Read the model definition and answer for the solid it produces. Units are mm, in the model's axes. A direction names the side the tool comes from. Coordinates: 2 decimals unless noted, no trailing zeros. Loops run counter-clockwise (first coordinate to the right, second up) from the corner with the lowest first, then second, coordinate; pieces in that order, holes last. Notation, with made-up numbers: (74, 76.25) - (115, 76.25) arc R30 ccw to (115, 112.25) - close; hole circle Ø10 at (-11.5, 47.5). An arc over 180 degrees is marked (long way). Use one line per item in the form item = value.
Autodesk Inventor part; units mm, degrees
ref_plane "YZ Plane" through (0, 0, 0) normal (1, 0, 0) x (0, 1, 0)
ref_plane "XZ Plane" through (0, 0, 0) normal (0, 1, 0) x (-1, 0, 0)
ref_plane "XY Plane" through (0, 0, 0) normal (0, 0, 1) x (1, 0, 0)
sketch "Sketch1" plane through (0, 0, 0) normal (0, 0, 1) x (1, 0, 0)
  line L0 (-11, 11) -> (11, 11)
  line L1 (11, 11) -> (11, -11)
  line L2 (11, -11) -> (-11, -11)
  line L3 (-11, -11) -> (-11, 11)
  point P0 (0, 0)
  point P1 (-11, 0)
  point P2 (0, 11)
  dimension "d0" = 22
extrude "Extrusion1" add sketch "Sketch1" along normal blind 3.4
sketch "Sketch2" plane through (0, 0, 3.4) normal (0, 0, 1) x (1, 0, 0)
  circle A0 centre (0, 0) radius 8.98 construction
  line L0 (-6.3498, 6.3498) -> (6.3498, 6.3498) construction
  line L1 (6.3498, 6.3498) -> (6.3498, -6.3498) construction
  line L2 (6.3498, -6.3498) -> (-6.3498, -6.3498) construction
  line L3 (-6.3498, -6.3498) -> (-6.3498, 6.3498) construction
  line L4 (-3.4498, 8.0241) -> (-3.4498, 4.6755)
  line L5 (-3.4498, 4.6755) -> (-6.3498, 3.0012)
  line L6 (-6.3498, 3.0012) -> (-9.2498, 4.6755)
  line L7 (-9.2498, 4.6755) -> (-9.2498, 8.0241)
  line L8 (-9.2498, 8.0241) -> (-6.3498, 9.6985)
  line L9 (-6.3498, 9.6985) -> (-3.4498, 8.0241)
  line L10 (9.2498, 8.0241) -> (9.2498, 4.6755)
  line L11 (9.2498, 4.6755) -> (6.3498, 3.0012)
  line L12 (6.3498, 3.0012) -> (3.4498, 4.6755)
  line L13 (3.4498, 4.6755) -> (3.4498, 8.0241)
  line L14 (3.4498, 8.0241) -> (6.3498, 9.6985)
  line L15 (6.3498, 9.6985) -> (9.2498, 8.0241)
  line L16 (9.2498, -4.6755) -> (9.2498, -8.0241)
  line L17 (9.2498, -8.0241) -> (6.3498, -9.6985)
  line L18 (6.3498, -9.6985) -> (3.4498, -8.0241)
  line L19 (3.4498, -8.0241) -> (3.4498, -4.6755)
  line L20 (3.4498, -4.6755) -> (6.3498, -3.0012)
  line L21 (6.3498, -3.0012) -> (9.2498, -4.6755)
  line L22 (-6.3498, -3.0012) -> (-3.4498, -4.6755)
  line L23 (-3.4498, -4.6755) -> (-3.4498, -8.0241)
  line L24 (-3.4498, -8.0241) -> (-6.3498, -9.6985)
  line L25 (-6.3498, -9.6985) -> (-9.2498, -8.0241)
  line L26 (-9.2498, -8.0241) -> (-9.2498, -4.6755)
  line L27 (-9.2498, -4.6755) -> (-6.3498, -3.0012)
  point P0 (6.3498, -6.3498)
  dimension "d3" = 17.96
  dimension "d4" = 5.8
extrude "Extrusion2" cut sketch "Sketch2" against normal blind 4
sketch "Sketch3" plane through (0, 0, 0) normal (0, 0, -1) x (-1, 0, 0)
  line L0 (-3.4498, -4.6755) -> (-3.4498, -8.0241)
  line L1 (-3.4498, -8.0241) -> (-6.3498, -9.6985)
  line L2 (-6.3498, -9.6985) -> (-9.2498, -8.0241)
  line L3 (-9.2498, -8.0241) -> (-9.2498, -4.6755)
  line L4 (-9.2498, -4.6755) -> (-6.3498, -3.0012)
  line L5 (-6.3498, -3.0012) -> (-3.4498, -4.6755)
  line L6 (-3.4498, 8.0241) -> (-3.4498, 4.6755)
  line L7 (-3.4498, 4.6755) -> (-6.3498, 3.0012)
  line L8 (-6.3498, 3.0012) -> (-9.2498, 4.6755)
  line L9 (-9.2498, 4.6755) -> (-9.2498, 8.0241)
  line L10 (-9.2498, 8.0241) -> (-6.3498, 9.6985)
  line L11 (-6.3498, 9.6985) -> (-3.4498, 8.0241)
  line L12 (9.2498, -8.0241) -> (6.3498, -9.6985)
  line L13 (6.3498, -9.6985) -> (3.4498, -8.0241)
  line L14 (3.4498, -8.0241) -> (3.4498, -4.6755)
  line L15 (3.4498, -4.6755) -> (6.3498, -3.0012)
  line L16 (6.3498, -3.0012) -> (9.2498, -4.6755)
  line L17 (9.2498, -4.6755) -> (9.2498, -8.0241)
  line L18 (9.2498, 8.0241) -> (9.2498, 4.6755)
  line L19 (9.2498, 4.6755) -> (6.3498, 3.0012)
  line L20 (6.3498, 3.0012) -> (3.4498, 4.6755)
  line L21 (3.4498, 4.6755) -> (3.4498, 8.0241)
  line L22 (3.4498, 8.0241) -> (6.3498, 9.6985)
  line L23 (6.3498, 9.6985) -> (9.2498, 8.0241)
  line L24 (11, -11) -> (-11, -11)
  line L25 (11, 11) -> (11, -11)
  line L26 (-11, 11) -> (11, 11)
  line L27 (-11, -11) -> (-11, 11)
  circle A0 centre (6.3498, 6.3498) radius 1.75
  circle A1 centre (6.3498, -6.3498) radius 1.75
  circle A2 centre (-6.3498, -6.3498) radius 1.75
  circle A3 centre (-6.3498, 6.3498) radius 1.75
  point P0 (0, 0)
  point P1 (9.2498, -6.3498)
  point P2 (-3.4498, -6.3498)
  point P3 (-3.4498, 6.3498)
  point P4 (9.2498, 6.3498)
  dimension "d7" = 3.5
extrude "Extrusion3" add sketch "Sketch3" against normal blind 1 contours L0 L1 L2 L3 L4 L5 | L6 L7 L8 L9 L10 L11 | L12 L13 L14 L15 L16 L17 | L18 L19 L20 L21 L22 L23
fillet "Fillet1" radius 2 4 edges at (11, 11, 1.7) (-11, 11, 1.7) (11, -11, 1.7) (-11, -11, 1.7)
sketch "Sketch4" plane through (0, 0, 3.4) normal (0, 0, 1) x (1, 0, 0)
  circle A0 centre (0, 0) radius 4.1
  dimension "d11" = 8.2
extrude "Extrusion4" cut sketch "Sketch4" against normal through all
chamfer "Chamfer1" distance 0.4 angle 45 16 edges at (0, 11, 0) (-10.4142, 10.4142, 0) (-11, 0, 0) (-10.4142, -10.4142, 0) (0, -11, 0) (10.4142, -10.4142, 0) (11, 0, 0) (10.4142, 10.4142, 0) (0, 11, 3.4) (-10.4142, 10.4142, 3.4) (-11, 0, 3.4) (-10.4142, -10.4142, 3.4) (0, -11, 3.4) (10.4142, -10.4142, 3.4) (11, 0, 3.4) (10.4142, 10.4142, 3.4)
chamfer "Chamfer2" distance 0.4 angle 45 2 edges at (-4.1, 0, 0) (-4.1, 0, 3.4)
properties part number "bnc-nut-support" material "ABS Plastic"
Item 1: The part is cut by section A-A on y = 0. Give the vertices of the cut face in (x, z).
Results below:
outline = (-11, 0.4) - (-10.6, 0) - (-4.5, 0) - (-4.1, 0.4) - (-4.1, 3) - (-4.5, 3.4) - (-10.6, 3.4) - (-11, 3) - close; (4.1, 0.4) - (4.5, 0) - (10.6, 0) - (11, 0.4) - (11, 3) - (10.6, 3.4) - (4.5, 3.4) - (4.1, 3) - close
Item 2: Find the intervals of material crossed by L1, parallel to X at y = 7, z = 2.8; L2, parallel to X at y = -6.5, z = 0.85; L3, parallel to Y at x = -6, z = 2.45, in increasing order.
Results below:
L1 = -11 to -9.25, -3.45 to 3.45, 9.25 to 11
L2 = -11 to -8.09, -4.61 to 4.61, 8.09 to 11
L3 = -11 to -9.5, -3.2 to 3.2, 9.5 to 11
Item 3: The part is cut by section D-D on y = 7. Give the vertices of the cut face in (x, z).
Results below:
outline = (-11, 0.4) - (-10.6, 0) - (-7.97, 0) - (-7.97, 1) - (-9.25, 1) - (-9.25, 3.4) - (-10.6, 3.4) - (-11, 3) - close; (-4.73, 0) - (4.73, 0) - (4.73, 1) - (3.45, 1) - (3.45, 3.4) - (-3.45, 3.4) - (-3.45, 1) - (-4.73, 1) - close; (7.97, 0) - (10.6, 0) - (11, 0.4) - (11, 3) - (10.6, 3.4) - (9.25, 3.4) - (9.25, 1) - (7.97, 1) - close
Item 4: The part is cut by section C-C on z = 2.5. Count the separate pieces of the cut face and the enclosed holes in it, plus the area to 3 significant figures.
Results below:
separate_pieces = 1
enclosed_holes = 5
area = 311 mm²
Item 5: For a pull along Y with two mould halves and no side action, classify faces 3 (the flat face through (-4.88, -8.85, 2.22)), 4 (the flat face through (-7.779, 3.827, 2.217)), 5 (the flat face through (11, 0, 2)), 6 (the conical face through (10.225, -10.199, 3.286)) as +Y half, -Y half, draft (parallel to the pull), parting line (faces both ways), or undercut.
Results below:
face_3 = undercut
face_4 = undercut
face_5 = draft
face_6 = -Y half
Item 6: Each of these flat-tipped pins is pushed along its axis until it touches: P1, Ø1.5, axis at x = 5, y = -8.5, coming from the +Z side; P2, Ø1.7, axis at x = -7.5, y = -7.5, coming from the +Z side. Where does it stop, or does it pass through?
Results below:
P1 = 3.4
P2 = 1
Item 7: Which of the six approach directions +Z, -Z, +X, -X, +Y, -Y give full straight-line access (tool end or side, diameter ignored) to faces 1 (the flat face through (7.82, -8.85, 2.22)), 2 (the conical face through (-10.199, -10.225, 3.286))?
Results below:
face_1 = +Z
face_2 = +Z, -X, -Y
